from build123d import *

# Parameters (mm, degrees)
BOSS_EXTRUDE1_DEPTH = 12


with BuildPart() as part:
    # Sketch1 → Boss-Extrude1 (new body)
    with BuildSketch(Plane(origin=(0, 0, 0), x_dir=(1, 0, 0), z_dir=(0, 1, 0))):
        with BuildLine():
            Line((-420, 0), (-264.641016151, 0))
            ThreePointArc((-264.641016151, 0), (-255.980762114, 5), (-255.980762114, 15))
            ThreePointArc((-255.980762114, 15), (-255.980762114, 25), (-247.320508076, 30))
            Line((-247.320508076, 30), (-207.320508076, 30))
            ThreePointArc((-207.320508076, 30), (-198.660254038, 25), (-198.660254038, 15))
            ThreePointArc((-198.660254038, 15), (-198.660254038, 5), (-190, 0))
            Line((-190, 0), (-140, 0))
            ThreePointArc((-140, 0), (1.07e-06, 140), (140, -2.139e-06))
            Line((140, -2.139e-06), (190, -2.149e-06))
            ThreePointArc((190, -2.149e-06), (198.660254037, -5.000002151), (198.660254035, -15.000002151))
            ThreePointArc((198.660254035, -15.000002151), (198.660254033, -25.000002151), (207.32050807, -30.000002153))
            Line((207.32050807, -30.000002153), (247.32050807, -30.000002161))
            ThreePointArc((247.32050807, -30.000002161), (255.980762108, -25.000002163), (255.98076211, -15.000002163))
            ThreePointArc((255.98076211, -15.000002163), (255.980762113, -5.000002163), (264.641016151, -2.165e-06))
            Line((264.641016151, -2.165e-06), (420, -2.196e-06))
            ThreePointArc((420, -2.196e-06), (1.098e-06, 420), (-420, 0))
        make_face()
    extrude(amount=BOSS_EXTRUDE1_DEPTH)


solid = part.part
Build history of the part. All positions in model axes, mm. Give positions to 0.01 mm unless a question says otherwise; leave off trailing zeros. Loops run counter-clockwise (first coordinate to the right, second up) from the corner with the lowest first, then second, coordinate; pieces in that order, holes last. Notation, with made-up numbers: (-6, -35) - (43, -35) arc R26 ccw to (43, 2) - close; hole circle Ø8 at (-24, 81). An arc over 180 degrees is marked (long way). Write item = value, one per line. Start each with the question number.
1) Band-saw the part on A-A on z = -93.5. Give the cut face in (x, y), plus the area to 3 significant figures.
2) Band-saw the part on C-C on x = 0. Give the cut face in (y, z).
3) Probe probe 1 along X at (y, z) = (6.75, -7); probe 2 along X at (y, z) = (2, -332); probe 3 along X at (y, z) = (6.25, 11.5). List the from-to ranges inside material, lowest first. Write a range as from..to.
4) Band-saw the part on D-D on z = -386.5. Give the cut face in (x, y).
5) Pull direction X, two halves, no side cores. Call faces 1 (the flat face through (-6, 12, -198)), 2 (the cylindrical face through (-3.079, 5.916, -139.966)), 3 (the cylindrical face through (9.2, 5.9, -419.9)): +X half, -X half, draft (parallel to the pull), parting line (faces both ways), or undercut.
6) Band-saw the part on B-B on y = 5.75. Give the cut face in (x, z).
7) Drop flat-ended pins along their axis: pin 1 Ø4 at (y, z) = (8, -125) entering from -X; pin 2 Ø6 at (x, y) = (-323, 5) entering from +Z; pin 3 Ø2 at (x, y) = (-86.5, 3.5) entering from +Z. Give the stop position or say it passes through.
Final values:
q1.outline = (-409.46, 0) - (-104.2, 0) - (-104.2, 12) - (-409.46, 12) - close; (104.2, 0) - (409.46, 0) - (409.46, 12) - (104.2, 12) - close
q1.area = 7,330 mm²
q2.outline = (0, -420) - (12, -420) - (12, -140) - (0, -140) - close
q3.probe_1 = -419.94..-255.1, -199.54..-139.82, 139.82..419.94
q3.probe_2 = -257.25..257.25
q3.probe_3 = 199.89..254.75
q4.outline = (-164.37, 0) - (164.37, 0) - (164.37, 12) - (-164.37, 12) - close
q5.face_1 = draft
q5.face_2 = undercut
q5.face_3 = parting line
q6.outline = (-420, 0) arc R420 ccw to (420, 0) - (264.64, 0) arc R10 cw to (255.98, 15) arc R10 ccw to (247.32, 30) - (207.32, 30) arc R10 ccw to (198.66, 15) arc R10 cw to (190, 0) - (140, 0) arc R140 cw to (-140, 0) - (-190, 0) arc R10 ccw to (-198.66, -15) arc R10 cw to (-207.32, -30) - (-247.32, -30) arc R10 cw to (-255.98, -15) arc R10 ccw to (-264.64, 0) - close
q7.pin_1 = -401.59
q7.pin_2 = 0
q7.pin_3 = -109.29
